Geometry check sheet. Reference: the model listing, model coordinates, mm. Face numbers are marked on the shaded views. A direction names the side the tool comes from. Coordinates: 2 decimals unless noted, no trailing zeros. Write each loop counter-clockwise with the first axis right and the second up, starting at its lowest first coordinate (ties: lowest second). Pieces come first, ordered by that corner, then holes. Notation, with made-up numbers: (20.5, 14.5) -> (24.5, 14.5) arc R14 cw to (24.5, 34.5) -> close; hole circle Ø10 at (-8, 48.5). An arc over 180 degrees is marked (long way). Answer as CSV lines item,"result".
```python
from build123d import *

# Parameters (mm, degrees)
SKETCH1_W            = 50
SKETCH1_H            = 18
BOSS_EXTRUDE1_DEPTH  = 7
SKETCH2_W            = 50
SKETCH2_H            = 8
BOSS_EXTRUDE2_DEPTH  = 6.7
SKETCH3_W            = 7
SKETCH3_H            = 8
BOSS_EXTRUDE3_DEPTH  = 23
SKETCH4_W            = 7
SKETCH4_H            = 8
BOSS_EXTRUDE4_DEPTH  = 14
SKETCH5_W            = 50
SKETCH5_H            = 10
CUT_EXTRUDE1_DEPTH   = 14
SKETCH6_R            = 2
CUT_EXTRUDE2_DEPTH   = 14
SKETCH7_W            = 50
SKETCH7_H            = 6
BOSS_EXTRUDE5_DEPTH  = 67.91
CUT_EXTRUDE3_DEPTH   = 35
SKETCH9_R            = 2
CUT_EXTRUDE5_DEPTH   = 35
SKETCH13_W           = 14
SKETCH13_H           = 8
CUT_EXTRUDE6_DEPTH   = 10
SKETCH14_W           = 7.7
SKETCH14_H           = 8
CUT_EXTRUDE7_DEPTH   = 120
SKETCH15_W           = 50
SKETCH15_H           = 14
BOSS_EXTRUDE6_DEPTH  = 6.4
SKETCH16_W           = 50
SKETCH16_H           = 14
CUT_EXTRUDE8_DEPTH   = 6
BOSS_EXTRUDE7_DEPTH  = 50
SKETCH18_R           = 2
CUT_EXTRUDE9_DEPTH   = 6.4
SKETCH19_R           = 3.5
CUT_EXTRUDE10_DEPTH  = 6.4
SKETCH20_W           = 12.4
SKETCH20_H           = 26.067854841
CUT_EXTRUDE11_DEPTH  = 70
SKETCH21_W           = 50
SKETCH21_H           = 6
BOSS_EXTRUDE8_DEPTH  = 10
SKETCH22_W           = 50
SKETCH22_H           = 10
BOSS_EXTRUDE9_DEPTH  = 18.28
SKETCH23_W           = 50
SKETCH23_H           = 6
BOSS_EXTRUDE10_DEPTH = 14
SKETCH24_R           = 2
CUT_EXTRUDE12_DEPTH  = 14
BOSS_EXTRUDE11_DEPTH = 50
SKETCH26_R           = 3.5
CUT_EXTRUDE13_DEPTH  = 14
SKETCH27_W           = 16.816450925
SKETCH27_H           = 29.203857669
BOSS_EXTRUDE12_DEPTH = 6
SKETCH28_R           = 6.25
CUT_EXTRUDE14_DEPTH  = 10


with BuildPart() as part:
    # Sketch1 → Boss-Extrude1 (new body)
    with BuildSketch(Plane.XY):
        with Locations((-12.394067797, 1.955508475)):
            Rectangle(SKETCH1_W, SKETCH1_H)
    extrude(amount=BOSS_EXTRUDE1_DEPTH)

    # Sketch2 → Boss-Extrude2 (add)
    with BuildSketch(Plane.XY.offset(7)):
        with Locations((-12.394067797, 6.955508475)):
            Rectangle(SKETCH2_W, SKETCH2_H)
    extrude(amount=BOSS_EXTRUDE2_DEPTH)

    # Sketch3 → Boss-Extrude3 (add)
    with BuildSketch(Plane(origin=(12.605932203, 0, 0), x_dir=(0, 0, -1), z_dir=(1, 0, 0))):
        with Locations((-3.5, 6.955508475)):
            Rectangle(SKETCH3_W, SKETCH3_H)
    extrude(amount=BOSS_EXTRUDE3_DEPTH)

    # Sketch4 → Boss-Extrude4 (add)
    with BuildSketch(Plane.ZY.offset(37.394067797)):
        with Locations((3.5, 6.955508475)):
            Rectangle(SKETCH4_W, SKETCH4_H)
    extrude(amount=BOSS_EXTRUDE4_DEPTH)

    # Sketch5 → Cut-Extrude1 (cut)
    with BuildSketch(Plane.XY.offset(7)):
        with Locations((-12.394067797, -2.044491525)):
            Rectangle(SKETCH5_W, SKETCH5_H)
    extrude(amount=-CUT_EXTRUDE1_DEPTH, mode=Mode.SUBTRACT)

    # Sketch6 → Cut-Extrude2 (cut)
    with BuildSketch(Plane.XY.offset(7)):
        with Locations((19.605932203, 6.955508475)):
            Circle(SKETCH6_R)
        with Locations((28.605932203, 6.955508475)):
            Circle(SKETCH6_R)
    extrude(amount=-CUT_EXTRUDE2_DEPTH, mode=Mode.SUBTRACT)

    # Sketch7 → Boss-Extrude5 (add)
    with BuildSketch(Plane.XZ.offset(-2.955508475)):
        with Locations((-12.394067797, 10.7)):
            Rectangle(SKETCH7_W, SKETCH7_H)
    extrude(amount=BOSS_EXTRUDE5_DEPTH)

    # Sketch8 → Cut-Extrude3 (cut)
    with BuildSketch(Plane.XY.offset(13.7)):
        with BuildLine():
            Line((-4.394067797, -44.33115583), (-4.394067797, -64.954491525))
            ThreePointArc((-4.394067797, -64.954491525), (-12.394067797, -72.954491525), (-20.394067797, -64.954491525))
            Line((-20.394067797, -64.954491525), (-20.394067797, -44.33115583))
            ThreePointArc((-20.394067797, -44.33115583), (-12.394067797, -36.33115583), (-4.394067797, -44.33115583))
        make_face()
    extrude(amount=-CUT_EXTRUDE3_DEPTH, mode=Mode.SUBTRACT)

    # Sketch9 → Cut-Extrude5 (cut)
    with BuildSketch(Plane(origin=(0, 0, 7.7), x_dir=(-1, 0, 0), z_dir=(0, 0, -1))):
        with Locations((27.901028765, -41.756933891)):
            Circle(SKETCH9_R)
        with Locations((4.616687569, -28.370715783)):
            Circle(SKETCH9_R)
    extrude(amount=-CUT_EXTRUDE5_DEPTH, mode=Mode.SUBTRACT)

    # Sketch13 → Cut-Extrude6 (cut)
    with BuildSketch(Plane.XY.offset(7)):
        with Locations((-44.394067797, 6.955508475)):
            Rectangle(SKETCH13_W, SKETCH13_H)
    extrude(amount=-CUT_EXTRUDE6_DEPTH, mode=Mode.SUBTRACT)

    # Sketch14 → Cut-Extrude7 (cut)
    with BuildSketch(Plane.ZY.offset(37.394067797)):
        with Locations((3.85, 6.955508475)):
            Rectangle(SKETCH14_W, SKETCH14_H)
    extrude(amount=-CUT_EXTRUDE7_DEPTH, mode=Mode.SUBTRACT)

    # Sketch15 → Boss-Extrude6 (add)
    with BuildSketch(Plane(origin=(0, 0, 7.7), x_dir=(-1, 0, 0), z_dir=(0, 0, -1))):
        with Locations((12.394067797, 3.955508475)):
            Rectangle(SKETCH15_W, SKETCH15_H)
    extrude(amount=BOSS_EXTRUDE6_DEPTH)

    # Sketch16 → Cut-Extrude8 (cut)
    with BuildSketch(Plane.XY.offset(13.7)):
        with Locations((-12.394067797, 3.955508475)):
            Rectangle(SKETCH16_W, SKETCH16_H)
    extrude(amount=-CUT_EXTRUDE8_DEPTH, mode=Mode.SUBTRACT)


with BuildPart() as cut_extrude8_piece_1:
    # of the separate pieces the step leaves, piece 1, a body of its own (cut_extrude8_pieces)
    add(part.part.solids().sort_by_distance((-37.394067797, -64.954491525, 13.7))[0])



with BuildPart() as cut_extrude8_piece_2:
    # of the separate pieces the step leaves, piece 2, a body of its own (cut_extrude8_pieces)
    add(part.part.solids().sort_by_distance((12.605932203, 10.955508475, 7.7))[0])


with BuildPart() as cut_extrude8_piece_1_1:
    add(cut_extrude8_piece_1.part)

    add(cut_extrude8_piece_2.part)  # Boss-Extrude7 merges Cut-Extrude8 piece 2
    # Sketch17 → Boss-Extrude7 (add)
    with BuildSketch(Plane.ZY.offset(37.394067797)):
        Polygon((7.7, 10.955508475), (13.7, -3.044491525), (7.7, -3.044491525), align=None)
        Polygon((1.3, -3.044491525), (7.7, -14.780389578), (7.7, -3.044491525), align=None)
    extrude(amount=-BOSS_EXTRUDE7_DEPTH)

    # Sketch18 → Cut-Extrude9 (cut)
    with BuildSketch(Plane(origin=(0, 0, 1.3), x_dir=(-1, 0, 0), z_dir=(0, 0, -1))):
        with Locations((-5.605932203, 3.955508475)):
            Circle(SKETCH18_R)
        with Locations((30.394067797, 4.955341008)):
            Circle(SKETCH18_R)
    extrude(amount=-CUT_EXTRUDE9_DEPTH, mode=Mode.SUBTRACT)

    # Sketch19 → Cut-Extrude10 (cut)
    with BuildSketch(Plane(origin=(0, 0, 7.7), x_dir=(-1, 0, 0), z_dir=(0, 0, -1))):
        with Locations((30.394067797, 4.955341008)):
            Circle(SKETCH19_R)
        with Locations((-5.605932203, 3.955508475)):
            Circle(SKETCH19_R)
    extrude(amount=-CUT_EXTRUDE10_DEPTH, mode=Mode.SUBTRACT)

    # Sketch20 → Cut-Extrude11 (cut)
    with BuildSketch(Plane.ZY.offset(37.394067797)):
        with Locations((7.5, -2.078418946)):
            Rectangle(SKETCH20_W, SKETCH20_H)
    extrude(amount=-CUT_EXTRUDE11_DEPTH, mode=Mode.SUBTRACT)

    # Sketch21 → Boss-Extrude8 (add)
    with BuildSketch(Plane(origin=(0, -15.112346366, 0), x_dir=(1, 0, 0), z_dir=(0, 1, 0))):
        with Locations((-12.394067797, -10.7)):
            Rectangle(SKETCH21_W, SKETCH21_H)
    extrude(amount=BOSS_EXTRUDE8_DEPTH)

    # Sketch22 → Boss-Extrude9 (add)
    with BuildSketch(Plane(origin=(0, 0, 7.7), x_dir=(-1, 0, 0), z_dir=(0, 0, -1))):
        with Locations((12.394067797, -10.112346366)):
            Rectangle(SKETCH22_W, SKETCH22_H)
    extrude(amount=BOSS_EXTRUDE9_DEPTH)

    # Sketch23 → Boss-Extrude10 (add)
    with BuildSketch(Plane(origin=(0, -5.112346366, 0), x_dir=(1, 0, 0), z_dir=(0, 1, 0))):
        with Locations((-12.394067797, 7.58)):
            Rectangle(SKETCH23_W, SKETCH23_H)
    extrude(amount=BOSS_EXTRUDE10_DEPTH)

    # Sketch24 → Cut-Extrude12 (cut)
    with BuildSketch(Plane.XY.offset(-4.58)):
        with Locations((2.605932203, 1.887653634)):
            Circle(SKETCH24_R)
        with Locations((-27.394067797, 1.887653634)):
            Circle(SKETCH24_R)
    extrude(amount=-CUT_EXTRUDE12_DEPTH, mode=Mode.SUBTRACT)

    # Sketch25 → Boss-Extrude11 (add)
    with BuildSketch(Plane.ZY.offset(37.394067797)):
        Polygon((7.7, -15.112346366), (0, -15.112346366), (7.7, -22.812346366), align=None)
        Polygon((-4.58, -5.112346366), (4.56, -5.112346366), (-4.58, 8.887653634), align=None)
    extrude(amount=-BOSS_EXTRUDE11_DEPTH)

    # Sketch26 → Cut-Extrude13 (cut)
    with BuildSketch(Plane(origin=(0, 0, -4.58), x_dir=(-1, 0, 0), z_dir=(0, 0, -1))):
        with Locations((27.394067797, 1.887653634)):
            Circle(SKETCH26_R)
        with Locations((-2.605932203, 1.887653634)):
            Circle(SKETCH26_R)
    extrude(amount=-CUT_EXTRUDE13_DEPTH, mode=Mode.SUBTRACT)

    # Sketch27 → Boss-Extrude12 (add)
    with BuildSketch(Plane(origin=(0, 0, 7.7), x_dir=(-1, 0, 0), z_dir=(0, 0, -1))):
        with Locations((11.985842335, -50.352562691)):
            Rectangle(SKETCH27_W, SKETCH27_H)
    extrude(amount=-BOSS_EXTRUDE12_DEPTH)

    # Sketch28 → Cut-Extrude14 (cut)
    with BuildSketch(Plane(origin=(0, 0, 7.7), x_dir=(-1, 0, 0), z_dir=(0, 0, -1))):
        with Locations((12.354948295, -48.879390068)):
            Circle(SKETCH28_R)
    extrude(amount=-CUT_EXTRUDE14_DEPTH, mode=Mode.SUBTRACT)


solid = cut_extrude8_piece_1_1.part
```
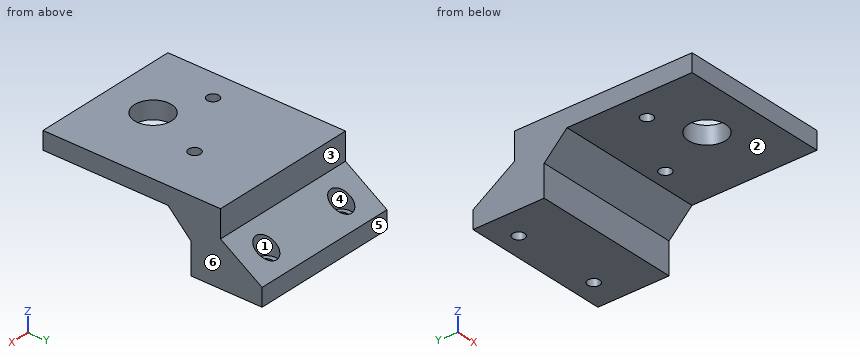
Item 1: Thickness scan on probe 1 along X at (y, z) = (2, -7); probe 2 along Z at (x, y) = (1, -33); probe 3 along Y at (x, z) = (5, 11). Record the ranges inside material, lowest first.
Responses:
probe 1,"x = -37.39 to -29.39, -25.4 to 0.61, 4.6 to 12.61"
probe 2,"z = 7.7 to 13.7"
probe 3,"y = -64.95 to -5.11"
Item 2: Cross-section at D-D, the plane x = -28.5. Record the cut outline in (y, z), plus the area to 3 significant figures.
Responses:
outline,"(-64.95, 7.7) -> (-43.67, 7.7) -> (-43.67, 13.7) -> (-64.95, 13.7) -> close; (-39.85, 7.7) -> (-22.81, 7.7) -> (-15.11, 0) -> (-15.11, -10.58) -> (0.22, -10.58) -> (0.22, -4.58) -> (-1.43, -4.58) -> (-1.43, 2.16) -> (-5.11, 4.56) -> (-5.11, 13.7) -> (-39.85, 13.7) -> close; (3.55, -10.58) -> (8.89, -10.58) -> (8.89, -4.58) -> (5.21, -2.18) -> (5.21, -4.58) -> (3.55, -4.58) -> close"
area,"646 mm2"
Item 3: Cross-section at B-B, the plane y = -47. Record the cut outline in (x, z).
Responses:
outline,"(-37.39, 7.7) -> (-18.32, 7.7) -> (-18.32, 13.7) -> (-37.39, 13.7) -> close; (-6.39, 7.7) -> (12.61, 7.7) -> (12.61, 13.7) -> (-6.39, 13.7) -> close"
Item 4: Cross-section at A-A, the plane x = -23. Record the cut outline in (y, z).
Responses:
outline,"(-64.95, 7.7) -> (-22.81, 7.7) -> (-15.11, 0) -> (-15.11, -10.58) -> (8.89, -10.58) -> (8.89, -4.58) -> (-5.11, 4.56) -> (-5.11, 13.7) -> (-64.95, 13.7) -> close"
Item 5: Release check for a two-part mould opening along X. For the marked faces 4, 5 and 6 record: +X half, -X half, draft (parallel to the pull), parting line (faces both ways), or undercut.
Responses:
face 4,"undercut"
face 5,"draft"
face 6,"+X half"
Item 6: Cross-section at C-C, the plane z = 11.5. Record the cut outline in (x, y), plus the area to 3 significant figures.
Responses:
outline,"(-37.39, -64.95) -> (12.61, -64.95) -> (12.61, -5.11) -> (-37.39, -5.11) -> close; hole circle Ø4 at (-27.9, -41.76); hole circle Ø12.5 at (-12.35, -48.88); hole circle Ø4 at (-4.62, -28.37)"
area,"2,840 mm2"
Item 7: Set-up check for the marked faces 1, 2 and 3: record each of +Z, -Z, +X, -X, +Y, -Y from which the full face is reachable in a straight line by a thin tool's end or side.
Responses:
face 1,"+Z"
face 2,"-Z, +X, -X, -Y"
face 3,"+Z, +X, -X, +Y"
Item 8: Depth check by flat-ended pin: pin 1 Ø2.5 at (x, z) = (-1.5, 9) entering from +Y; pin 2 Ø5.5 at (x, z) = (-21.5, -5.5) entering from -Y; pin 3 Ø6.5 at (x, y) = (2.61, 1.89) entering from +Z; pin 4 Ø5 at (y, z) = (-49.5, 7) entering from -X. Enter the tip coordinate at first touch or a pass-through.
Responses:
pin 1,"stops at y = -5.11"
pin 2,"stops at y = -15.11"
pin 3,"stops at z = -4.58"
pin 4,"stops at x = -37.39"
